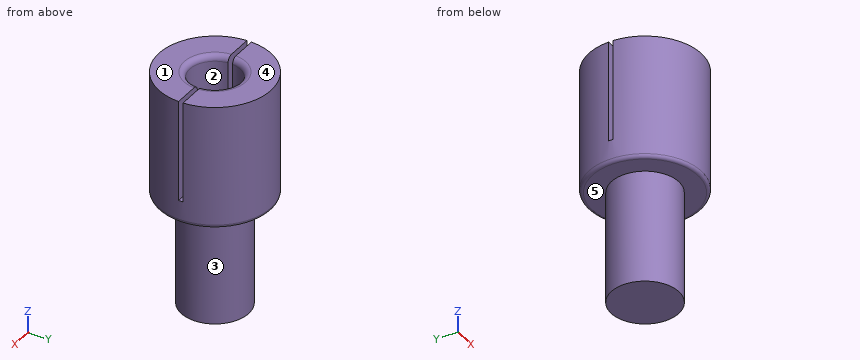
```python
from build123d import *

# Parameters (mm, degrees)
ESBO_O1_R                = 5
RESSALTO_EXTRUS_O1_DEPTH = 11
ESBO_O2_R                = 2.25
CORTE_EXTRUS_O1_DEPTH    = 11
ESBO_O3_R                = 3
RESSALTO_EXTRUS_O2_DEPTH = 10
CORTE_EXTRUS_O2_DEPTH    = 9
FILETE1_R                = 0.5
FILETE2_R                = 0.3


with BuildPart() as part:
    # Esboço1 → Ressalto-extrusão1 (new body)
    with BuildSketch(Plane.XY):
        with Locations((-26.183327478, 4.383756345)):
            Circle(ESBO_O1_R)
    extrude(amount=RESSALTO_EXTRUS_O1_DEPTH)

    # Esboço2 → Corte-extrusão1 (cut)
    with BuildSketch(Plane.XY.offset(11)):
        with Locations((-26.183327478, 4.383756345)):
            Circle(ESBO_O2_R)
    extrude(amount=-CORTE_EXTRUS_O1_DEPTH, mode=Mode.SUBTRACT)

    # Esboço3 → Ressalto-extrusão2 (add)
    with BuildSketch(Plane(origin=(0, 0, 0), x_dir=(-1, 0, 0), z_dir=(0, 0, -1))):
        with Locations(Location((26.183327478, 4.383756345, 0), (0, 0, 180))):
            Circle(ESBO_O3_R)
    extrude(amount=RESSALTO_EXTRUS_O2_DEPTH)

    # Esboço4 → Corte-extrusão2 (cut)
    with BuildSketch(Plane.XY.offset(11)):
        with BuildLine():
            Line((-31.183327478, 4.583756345), (-21.183327478, 4.583756345))
            ThreePointArc((-21.183327478, 4.583756345), (-20.983327478, 4.383756345), (-21.183327478, 4.183756345))
            Line((-21.183327478, 4.183756345), (-31.183327478, 4.183756345))
            ThreePointArc((-31.183327478, 4.183756345), (-31.383327478, 4.383756345), (-31.183327478, 4.583756345))
        make_face()
    extrude(amount=-CORTE_EXTRUS_O2_DEPTH, mode=Mode.SUBTRACT)

    # Filete1
    filete1_edges = [part.edges().sort_by_distance(p)[0] for p in [
        (-26.183327478, 2.133756345, 11),
        (-26.183327478, 6.633756345, 11),
    ]]
    fillet(filete1_edges, radius=FILETE1_R)

    # Filete2
    filete2_edges = [part.edges().sort_by_distance(p)[0] for p in [
        (-31.183327478, 4.383756345, 0),
    ]]
    fillet(filete2_edges, radius=FILETE2_R)


solid = part.part
```
Model file for the job. Use its own axes, mm. Face numbers are marked on the shaded views. A direction names the side the tool comes from. Coordinates: 2 decimals unless noted, no trailing zeros. Loops run counter-clockwise (first coordinate to the right, second up) from the corner with the lowest first, then second, coordinate; pieces in that order, holes last. Notation, with made-up numbers: M 14,44 L 36,44 A20 ccw 36,68 Z; hole C -11,84.25 d9. An arc over 180 degrees is marked long. Use CSV: the item, a comma, the result in double quotes. Start each with the question number.
1. Band-saw the part on A-A, the plane z = 9.75. List the corners of the cut face in (x, y).
2. Two-plate mould, pull along X, no slides. Class the marked faces 1, 2 and 3: pulls with the +X half, pulls with the -X half, needs draft (parallel to the pull), parting line crosses it, or undercut.
3. Tool access for the marked faces 4 and 5: list every direction of +Z, -Z, +X, -X, +Y, -Y with a clear straight run to the whole face (end or side of a thin tool).
4. Probe probe 1 along Z at (x, y) = (-22.75, 5.5); probe 2 along Y at (x, z) = (-26, -4); probe 3 along Y at (x, z) = (-22.5, 7.5). List the from-to ranges inside material, lowest first. Write a range as [from, to].
5. Band-saw the part on B-B, the plane z = -8. List the corners of the cut face in (x, y).
6. Flat gauge pins, fed straight in: pin 1 (1.5 mm diameter, centred on y = 4.5, z = -3.5, fed in from -X); pin 2 (1.3 mm diameter, centred on x = -26, y = 5.5, fed in from +Z); pin 3 (4 mm diameter, centred on x = -27.5, z = -4.5, fed in from +Y). Where does each tip first touch, or does it go through?
Entries:
1,outline,"M -31.18,4.18 A5 ccw -21.19,4.18 L -23.94,4.18 A2.25 cw -28.42,4.18 Z; M -31.18,4.58 L -28.42,4.58 A2.25 cw -23.94,4.58 L -21.19,4.58 A5 ccw Z"
2,face 1,"needs draft"
2,face 2,"undercut"
2,face 3,"parting line crosses it"
3,face 4,"+Z, +X, -X, +Y, -Y"
3,face 5,"-Z"
4,probe 1,"z = [0, 11]"
4,probe 2,"y = [1.39, 7.38]"
4,probe 3,"y = [1, 4.18], [4.58, 7.77]"
5,outline,"C -26.18,4.38 d6"
6,pin 1,"stops at x = -29.18"
6,pin 2,"stops at z = 0"
6,pin 3,"stops at y = 7.38"
